Input: part model. Units: mm. Frame: model coordinates. A direction names the side the tool comes from. Coordinates: 2 decimals unless noted, no trailing zeros. Write each loop counter-clockwise with the first axis right and the second up, starting at its lowest first coordinate (ties: lowest second). Pieces come first, ordered by that corner, then holes.
1) Set-up query: faces 1 (the flat face through (175.61, -0.99, 260.5)), 2 (the cylindrical face through (-242.06, -1.014, -129.913)). Return all of +Z, -Z, +X, -X, +Y, -Y with unobstructed straight access to the full face (end or side cutting, diameter ignored); none if empty.
2) Section query B-B (z = 92). Output: boundary loops of the cut face in (x, y), then the cut area to 3 significant figures.
3) Line query: L1, parallel to Z at x = 5, y = -0.4; L2, parallel to X at y = -0.55, z = -85; L3, parallel to Y at x = -170, z = -156.5. Output: solid intervals per line, ascending.
4) Draft query along Z for faces 3 (the flat face through (-281.6, -1, 261.9)), 4 (the flat face through (-57, 0, 231)), 5 (the cylindrical face through (135.4, -1, 195.1)), 6 (the cylindrical face through (134.58, -1.01, -130.7)). Return one class per face: pulls with the +Z half, pulls with the -Z half, needs draft (parallel to the pull), parting line crosses it, or undercut.
5) Pin query (flat end, axial travel): pin 1 Ø7.5 at (x, z) = (-294.85, 7.21) entering from +Y; pin 2 Ø4 at (x, z) = (188.15, 185.01) entering from +Y; pin 3 Ø0.5 at (y, z) = (0.5, 249.5) entering from -X. Return the tip coordinate at first contact, or that it passes through.
6) Section query A-A (x = -59). Output: boundary loops of the cut face in (y, z).
7) Section query C-C (y = -0.55). Output: boundary loops of the cut face in (x, z), then the cut area to 3 significant figures.
from build123d import *

# Parameters (mm, degrees)
F1_DEPTH = 2
F3_DEPTH = 2.001
F4_W     = 3
F4_H     = 69.7761774063
F5_DEPTH = 3
F7_D     = 6.6


with BuildPart() as f1:
    # F0 (on Front) → F1 (new body)
    with BuildSketch(Plane.XZ):
        Polygon((-307.3464844827, 210.4111198679), (-307.3464844827, -195.9888801321), (200.6535155173, -195.9888801321), (200.6535155173, 210.4111198679), (149.8535155173, 312.0111198679), (-256.5464844827, 312.0111198679), align=None)
    extrude(amount=F1_DEPTH)

    # F2 (on face) → F3 (cut, through all)
    with BuildSketch(Plane.XZ.offset(2)):
        with BuildLine():
            Line((99.0535155173, 210.4111198679), (-205.7464844827, 210.4111198679))
            ThreePointArc((-205.7464844827, 210.4111198679), (-241.667508967, 195.5321443521), (-256.5464844827, 159.6111198679))
            Line((-256.5464844827, 159.6111198679), (-256.5464844827, -94.3888801321))
            ThreePointArc((-256.5464844827, -94.3888801321), (-241.667508967, -130.3099046164), (-205.7464844827, -145.1888801321))
            Line((-205.7464844827, -145.1888801321), (99.0535155173, -145.1888801321))
            ThreePointArc((99.0535155173, -145.1888801321), (134.9745400016, -130.3099046164), (149.8535155173, -94.3888801321))
            Line((149.8535155173, -94.3888801321), (149.8535155173, 159.6111198679))
            ThreePointArc((149.8535155173, 159.6111198679), (134.9745400016, 195.5321443521), (99.0535155173, 210.4111198679))
        make_face()
    extrude(amount=-F3_DEPTH, mode=Mode.SUBTRACT)

    # F4 (on face) → F5 (join)
    with BuildSketch(Plane.XZ.offset(2)):
        with Locations((-21.4731446389, 260.3619992733)):
            Rectangle(F4_W, F4_H)
    extrude(amount=-F5_DEPTH)

    # F7 (through all)
    with Locations(Plane.XZ.offset(2)):
        with Locations((-294.8464844827, 185.0111198679), (-294.8464844827, 7.2111198679), (-294.8464844827, -170.5888801321), (188.1535155173, -170.5888801321), (188.1535155173, 7.2111198679), (188.1535155173, 185.0111198679)):
            Hole(F7_D / 2)


solid = f1.part
Answer:
1. face 1: +Z, +X, +Y, -Y
1. face 2: +Y, -Y
2. outline: (-307.35, -2) - (-256.55, -2) - (-256.55, 0) - (-307.35, 0) - close; (149.85, -2) - (200.65, -2) - (200.65, 0) - (149.85, 0) - close
2. area: 203 mm2
3. L1: z = -195.99 to -145.19, 210.41 to 312.01
3. L2: x = -307.35 to -256.55, 149.85 to 200.65
3. L3: y = -2 to 0
4. face 3: pulls with the +Z half
4. face 4: needs draft
4. face 5: undercut
4. face 6: undercut
5. pin 1: stops at y = 0
5. pin 2: passes through
5. pin 3: stops at x = -22.97
6. outline: (-2, -195.99) - (0, -195.99) - (0, -145.19) - (-2, -145.19) - close; (-2, 210.41) - (0, 210.41) - (0, 312.01) - (-2, 312.01) - close
7. outline: (-307.35, -195.99) - (200.65, -195.99) - (200.65, 210.41) - (149.85, 312.01) - (-256.55, 312.01) - (-307.35, 210.41) - close; hole circle Ø6.6 at (-294.85, -170.59); hole circle Ø6.6 at (-294.85, 7.21); hole circle Ø6.6 at (-294.85, 185.01); hole (-256.55, -94.39) arc R50.8 ccw to (-205.75, -145.19) - (99.05, -145.19) arc R50.8 ccw to (149.85, -94.39) - (149.85, 159.61) arc R50.8 ccw to (99.05, 210.41) - (-205.75, 210.41) arc R50.8 ccw to (-256.55, 159.61) - close; hole circle Ø6.6 at (188.15, -170.59); hole circle Ø6.6 at (188.15, 7.21); hole circle Ø6.6 at (188.15, 185.01)
7. area: 110,000 mm2
